from build123d import *

# Parameters (mm, degrees)
SKETCH1_R               = 21
BOSS_EXTRUDE1_DEPTH     = 3
CUT_EXTRUDE1_DEPTH      = 30.849623113
CUT_EXTRUDE1_DEPTH_BACK = 30.849623113
SKETCH2_R               = 2.5
CUT_EXTRUDE2_DEPTH      = 30.849623113
CIRPATTERN1_COUNT       = 22
SKETCH4_W               = 7
SKETCH4_H               = 30.5
BOSS_EXTRUDE2_DEPTH     = 3
FILLET1_R               = 3
CUT_EXTRUDE3_DEPTH      = 48.947888379
CUT_EXTRUDE3_DEPTH_BACK = 48.947888379
SKETCH5_R               = 1.5


with BuildPart() as part:
    # Sketch1 → Boss-Extrude1 (new body)
    with BuildSketch(Plane(origin=(0, 0, 0), x_dir=(1, 0, 0), z_dir=(0, 1, 0))):
        with Locations(Location((0, 0, 0), (0, 0, 270))):
            Circle(SKETCH1_R)
    extrude(amount=BOSS_EXTRUDE1_DEPTH)

    # Sketch2 → Cut-Extrude1 (cut, two sides: drawn at the far end of the back side and taken through both)
    with BuildSketch(Plane(origin=(0, 3, 0), x_dir=(1, 0, 0), z_dir=(0, 1, 0)).offset(-CUT_EXTRUDE1_DEPTH_BACK)):
        with Locations(Location((0, 0, 0), (0, 0, 270))):
            Circle(SKETCH2_R)
    extrude(amount=CUT_EXTRUDE1_DEPTH + CUT_EXTRUDE1_DEPTH_BACK, mode=Mode.SUBTRACT)

    # Sketch3 → Cut-Extrude2 (cut, symmetric)
    with BuildSketch(Plane(origin=(0, 3, 0), x_dir=(1, 0, 0), z_dir=(0, 1, 0))):
        with BuildLine():
            Line((0.35, 14.3), (-0.35, 14.3))
            ThreePointArc((-0.35, 14.3), (-0.439436957, 14.337046001), (-0.476482958, 14.426482958))
            ThreePointArc((-0.476482958, 14.426482958), (-0.994323602, 17.794147764), (-2.5, 20.850659462))
            ThreePointArc((-2.5, 20.850659462), (0, 21), (2.5, 20.850659462))
            ThreePointArc((2.5, 20.850659462), (0.994323602, 17.794147764), (0.476482958, 14.426482958))
            ThreePointArc((0.476482958, 14.426482958), (0.439436957, 14.337046001), (0.35, 14.3))
        make_face()
    cut_extrude2 = extrude(amount=CUT_EXTRUDE2_DEPTH, both=True, mode=Mode.SUBTRACT)

    # CirPattern1: Cut-Extrude2 ×22 about axis
    cirpattern1_axis = Axis((0, 0, 0), (0, 1, 0))
    for i in range(1, CIRPATTERN1_COUNT):
        add(cut_extrude2.rotate(cirpattern1_axis, i * 360 / CIRPATTERN1_COUNT), mode=Mode.SUBTRACT)

    # Sketch4 → Boss-Extrude2 (add)
    with BuildSketch(Plane(origin=(0, 3, 0), x_dir=(1, 0, 0), z_dir=(0, 1, 0))):
        with Locations((0, 27.75)):
            Rectangle(SKETCH4_W, SKETCH4_H)
    extrude(amount=-BOSS_EXTRUDE2_DEPTH)

    # Fillet1
    fillet1_edges = [part.edges().sort_by_distance(p)[0] for p in [
        (3.5, 1.5, -43),
        (-3.5, 1.5, -43),
    ]]
    fillet(fillet1_edges, radius=FILLET1_R)

    # Sketch5 → Cut-Extrude3 (cut, two sides: drawn at the far end of the back side and taken through both)
    with BuildSketch(Plane(origin=(0, 3, 0), x_dir=(1, 0, 0), z_dir=(0, 1, 0)).offset(-CUT_EXTRUDE3_DEPTH_BACK)):
        with Locations(Location((0, 40, 0), (0, 0, 270))):
            Circle(SKETCH5_R)
    extrude(amount=CUT_EXTRUDE3_DEPTH + CUT_EXTRUDE3_DEPTH_BACK, mode=Mode.SUBTRACT)


solid = part.part
The model under review builds one solid part; all positions refer to its coordinate system, in mm. A direction names the side the tool comes from. Coordinates: 2 decimals unless noted, no trailing zeros. Write each loop counter-clockwise with the first axis right and the second up, starting at its lowest first coordinate (ties: lowest second). Pieces come first, ordered by that corner, then holes. Notation, with made-up numbers: (2.25, -27) -> (17.25, -27) arc R17 cw to (17.25, -20) -> close; hole circle Ø6 at (88, 57.5). An arc over 180 degrees is marked (long way). Answer in a Markdown table with one row per item.
1. Wall thickness on probe 1 along Z at (x, y) = (0, 0.8); probe 2 along Z at (x, y) = (13.5, 0.25); probe 3 along X at (y, z) = (1.65, 0): over which ranges is each line inside the solid? List them lowest first. Write a range as [from, to].
Answers below:
| item | result |
|---|---|
| probe 1 | z = [-43, -41.5], [-38.5, -2.5], [2.5, 14.3] |
| probe 2 | z = [-16.09, -13.74], [-10.62, -6.71], [-5.64, 5.64], [6.71, 10.62], [13.74, 16.09] |
| probe 3 | x = [-21, -2.5], [2.5, 21] |
2. Clearance check with flat-ended pins moving along their axes: pin 1 Ø1.5 at (y, z) = (1.5, -29.5) entering from -X; pin 2 Ø1 at (y, z) = (1.5, -31) entering from +X. State where each tip first meets the part, or that it passes through.
Answers below:
| item | result |
|---|---|
| pin 1 | stops at x = -3.5 |
| pin 2 | stops at x = 3.5 |
3. We need section B-B, the plane x = 15. State the section outline as (y, z) points.
Answers below:
| item | result |
|---|---|
| outline | (0, -11.25) -> (3, -11.25) -> (3, -7.66) -> (0, -7.66) -> close; (0, -6.17) -> (3, -6.17) -> (3, -2.67) -> (0, -2.67) -> close; (0, -1.66) -> (3, -1.66) -> (3, 1.66) -> (0, 1.66) -> close; (0, 2.67) -> (3, 2.67) -> (3, 6.17) -> (0, 6.17) -> close; (0, 7.66) -> (3, 7.66) -> (3, 11.25) -> (0, 11.25) -> close |
4. We need section A-A, the plane x = -16. State the section outline as (y, z) points, and give its area (3 significant figures).
Answers below:
| item | result |
|---|---|
| outline | (0, -11.53) -> (3, -11.53) -> (3, -8.51) -> (0, -8.51) -> close; (0, -6.4) -> (3, -6.4) -> (3, -2.93) -> (0, -2.93) -> close; (0, -1.7) -> (3, -1.7) -> (3, 1.7) -> (0, 1.7) -> close; (0, 2.93) -> (3, 2.93) -> (3, 6.4) -> (0, 6.4) -> close; (0, 8.51) -> (3, 8.51) -> (3, 11.53) -> (0, 11.53) -> close |
| area | 49.1 mm^2 |
5. Draft analysis for pull direction Z (two halves, no side actions). For faces 1 (the cylindrical face through (-2.64, 1.48, -42.1)), 2 (the cylindrical face through (15.81, 1.52, 8.33)), 3 (the flat face through (-3.5, 2, -30)), state which applies: +Z half, -Z half, draft (parallel to the pull), parting line (faces both ways), or undercut.
Answers below:
| item | result |
|---|---|
| face 1 | -Z half |
| face 2 | undercut |
| face 3 | draft |
6. For faces 4 (the flat face through (0, 0, -4)), 5 (the cylindrical face through (-17.428, 1.521, 3.496)), 6 (the cylindrical face through (8.796, 1.521, 15.553)), list the 3-axis set-ups (+Z, -Z, +X, -X, +Y, -Y) from which the entire face can be reached by the end or side of a thin tool; tool diameter is ignored.
Answers below:
| item | result |
|---|---|
| face 4 | +Z, -Z, +X, -X, -Y |
| face 5 | -X, +Y, -Y |
| face 6 | +Y, -Y |
7. We need section D-D, the plane z = 8. State the section outline as (x, y) points, and give its area (3 significant figures).
Answers below:
| item | result |
|---|---|
| outline | (-15.43, 0) -> (15.43, 0) -> (15.43, 3) -> (-15.43, 3) -> close |
| area | 92.6 mm^2 |
8. We need section C-C, the plane y = 2.5. Give the number of separate pieces and of enclosed holes in the cut face, and give its area (3 significant figures).
Answers below:
| item | result |
|---|---|
| separate pieces | 1 |
| enclosed holes | 2 |
| area | 1,190 mm^2 |
